Autodesk Inventor part; units mm, degrees
ref_plane "YZ Plane" through (0, 0, 0) normal (1, 0, 0) x (0, 1, 0)
ref_plane "XZ Plane" through (0, 0, 0) normal (0, 1, 0) x (-1, 0, 0)
ref_plane "XY Plane" through (0, 0, 0) normal (0, 0, 1) x (1, 0, 0)
sketch "Sketch1" plane through (0, 0, 0) normal (0, 1, 0) x (-1, 0, 0)
  line L0 (-275, 24.5536) -> (275, 24.5536)
  line L1 (275, 24.5536) -> (275, -24.5536)
  line L2 (275, -24.5536) -> (-275, -24.5536)
  line L3 (-275, -24.5536) -> (-275, 24.5536)
  point P0 (0, 0)
  dimension "d14" = 550
extrude "Extrusion1" add sketch "Sketch1" along normal mid plane 50
sketch "Sketch2" plane through (275, -25, -24.5536) normal (1, 0, 0) x (0, 0, -1)
  line L0 (0, 0) -> (0, 50)
  line L1 (0, 45) -> (-45, 45)
  line L2 (-45, 45) -> (-45, 0)
  line L3 (-49.1071, 0) -> (0, 0)
  line L4 (-45, 0) -> (0, 0)
  line L5 (0, 0) -> (0, 45)
  point P0 (-24.5536, 25)
extrude "Extrusion2" cut sketch "Sketch2" against normal through all
sketch "Sketch5" plane through (0, 25, 0) normal (0, 1, 0) x (1, 0, 0)
  line L0 (-275, 24.5536) -> (-275, -24.5536)
  line L1 (-275, 24.5536) -> (-225, 24.5536)
  line L2 (275, 24.5536) -> (-275, 24.5536)
  line L3 (-225, 24.5536) -> (-225, -20.4464)
  line L4 (-275, -20.4464) -> (275, -20.4464)
  line L5 (-225, -20.4464) -> (-275, -20.4464)
  line L6 (-275, -20.4464) -> (-275, 24.5536)
  line L7 (275, -24.5536) -> (275, 24.5536)
  line L8 (275, 24.5536) -> (225, 24.5536)
  line L9 (225, 24.5536) -> (225, -20.4464)
  line L10 (225, -20.4464) -> (275, -20.4464)
  line L11 (275, -20.4464) -> (275, 24.5536)
  point P0 (0, 0)
extrude "Extrusion5" cut sketch "Sketch5" against normal blind 10 contours L1 L3 L4 L0 | L2 L7 L4 L9
sketch "Sketch6" plane through (-275, 25, 24.5536) normal (0, 0, 1) x (1, 0, 0)
  line L0 (50, 0) -> (0, 0)
  line L1 (550, -50) -> (0, -50)
  line L2 (50, 0) -> (0, -50)
  line L3 (0, -50) -> (0, 0)
  line L4 (0, 0) -> (50, 0)
  line L5 (0, 0) -> (550, 0)
  line L6 (500, 0) -> (550, 0)
  line L7 (550, 0) -> (550, -50)
  line L8 (550, -50) -> (500, 0)
  point P0 (275, -25)
extrude "Extrusion6" cut sketch "Sketch6" against normal blind 5 contours L2 L3 L0 | L5 L7 L8
properties part number "angle1"
Input: part model. Units: mm. Frame: model coordinates. A direction names the side the tool comes from. Round coordinates to 2 decimals unless told otherwise and drop trailing zeros. Loops run counter-clockwise (first coordinate to the right, second up) from the corner with the lowest first, then second, coordinate; pieces in that order, holes last. Notation, with made-up numbers: (39.5, 36) - (71.5, 36) arc R13 ccw to (71.5, 46) - close; hole circle Ø8 at (-36.75, 19.25). An arc over 180 degrees is marked (long way). One line per item, written item: value. Start each with the question number.
(1) Contact query for flat-ended pins moving along their axis: P1, Ø22.5, axis at x = -29.5, z = 7, coming from the -Y side; P2, Ø1.5, axis at y = 22, z = 7, coming from the +X side; P3, Ø4, axis at y = 22, z = 9, coming from the -X side. Output: stop coordinate, or through.
(2) Section A-A, the plane x = 187. Return loops of the section in (y, z), plus the area to 3 significant figures.
(3) Ray query, line 1 (Y direction, x = 19.5, z = -8); line 2 (X direction, y = 21.5, z = -1.5); line 3 (Z direction, x = -195.5, y = -9). Return the intervals inside material, ascending. Write a range as [from, to].
(4) Draft query along Z for faces 3 (the flat face through (4, 0, 24.554)), 4 (the flat face through (3, 25, 0)). Return one class per face: +Z half, -Z half, draft (parallel to the pull), parting line (faces both ways), or undercut.
(5) Section B-B, the plane y = 4. Return loops of the section in (x, z), plus the area to 3 significant figures.
(6) Access query for faces 1 (the flat face through (250, 0, 23)), 2 (the flat face through (3, 20, -2)). Directions: +Z, -Z, +X, -X, +Y, -Y. A direction counts if a zero-diameter tool reaches every point of the face in a straight line with its end or side. Return the directions, or none.
(7) Section C-C, the plane z = -8.5. Return loops of the section in (x, y).
Results below:
1. P1: y = 20
1. P2: x = 225
1. P3: x = -225
2. outline: (-25, 20.45) - (20, 20.45) - (20, -24.55) - (25, -24.55) - (25, 24.55) - (-25, 24.55) - close
2. area: 430 mm^2
3. line 1: [20, 25]
3. line 2: [-225, 225]
3. line 3: [20.45, 24.55]
4. face 3: +Z half
4. face 4: draft
5. outline: (-246, 20.45) - (246, 20.45) - (246, 24.55) - (-246, 24.55) - close
5. area: 2,020 mm^2
6. face 1: +Z, -Z, +X, +Y
6. face 2: -Z, +X, -X, -Y
7. outline: (-225, 20) - (225, 20) - (225, 25) - (-225, 25) - close
